Model file for the job. Use its own axes, mm. A direction names the side the tool comes from. Coordinates: 2 decimals unless noted, no trailing zeros. Order: outer loops, then holes, each group sorted by start corner. A loop starts at its lowest first (then second) coordinate and runs counter-clockwise, first axis right, second up. Notation, with made-up numbers: (57.5, 85) -> (66.5, 85) arc R28 ccw to (66.5, 103) -> close; hole circle Ø8 at (65, 8.5). An arc over 180 degrees is marked (long way). Write item = value, one per line. Start each with the question number.
Q1. 3-axis set-ups, long thin cutter, end or side, ignore diameter. For faces 4 (the face through (-48, -66.033, 6)), 5 (the face through (63, -53.033, 2)), 6 (the face through (66.033, 47, 6)): which of +Z, -Z, +X, -X, +Y, -Y reach the whole face in a straight line?
Q2. Flat gauge pins, fed straight in: pin 1 (6 mm diameter, centred on y = 32.5, z = 5, fed in from +X); pin 2 (2.5 mm diameter, centred on x = -61.5, z = 1.5, fed in from +Y); pin 3 (6.5 mm diameter, centred on x = 61.5, y = 61.5, fed in from -Z). Where does each tip first touch, or does it go through?
Q3. Cut at A-A, the plane y = -28. List the corners of the cut face in (x, z), plus the area to 3 significant figures.
Q4. Cut at B-B, the plane x = 50.5. List the corners of the cut face in (y, z), plus the area to 3 significant figures.
Q5. Mould opens along Y. For faces 1 (the face through (-63, -53.033, 2)), 2 (the face through (-66.033, -47, 6)), 3 (the face through (61.15, -62.06, 7.46)) say: +Y half, -Y half, draft (parallel to the pull), parting line (faces both ways), or undercut.
Q6. Cut at C-C, the plane z = 2. Give the number of separate pieces and of enclosed holes in the cut face, plus the area to 3 significant figures.
Q7. Wall check: line 1 (X direction, y = 57.5, z = 9); line 2 (X direction, y = 58, z = 6); line 3 (Y direction, x = 17.3, z = 3.5) (3 decimals). Give the ranges that are in metal, low to high. Write a range as from..to.
Autodesk Inventor part; units mm, degrees
ref_plane "YZ Plane" through (0, 0, 0) normal (1, 0, 0) x (0, 1, 0)
ref_plane "XZ Plane" through (0, 0, 0) normal (0, 1, 0) x (-1, 0, 0)
ref_plane "XY Plane" through (0, 0, 0) normal (0, 0, 1) x (1, 0, 0)
sketch "Эскиз1" plane through (0, 0, 0) normal (0, 0, 1) x (1, 0, 0)
  circle A0 centre (59.533, -59.533) radius 3
  circle A1 centre (-59.533, -59.533) radius 3
  circle A2 centre (-59.533, 59.533) radius 3
  circle A3 centre (59.533, 59.533) radius 3
  circle A4 centre (0, 0) radius 65
  arc A5 (35.5618, 66.033) -> (-35.5618, 66.033) centre (0, 0) ccw
  line L0 (-35.5618, 66.033) -> (-66.033, 66.033)
  line L1 (-66.033, 66.033) -> (-66.033, 35.5618)
  arc A6 (-66.033, 35.5618) -> (-66.033, -35.5618) centre (0, 0) ccw
  line L2 (-66.033, -35.5618) -> (-66.033, -66.033)
  line L3 (-66.033, -66.033) -> (-35.5618, -66.033)
  arc A7 (-35.5618, -66.033) -> (35.5618, -66.033) centre (0, 0) ccw
  line L4 (35.5618, -66.033) -> (66.033, -66.033)
  line L5 (66.033, -66.033) -> (66.033, -35.5618)
  arc A8 (66.033, -35.5618) -> (66.033, 35.5618) centre (0, 0) ccw
  line L6 (66.033, 35.5618) -> (66.033, 66.033)
  line L7 (66.033, 66.033) -> (35.5618, 66.033)
  point P0 (0, 0)
extrude "Выдавливание1" add sketch "Эскиз1" along normal blind 10 contours A4 | L7 L6 A8 L5 L4 A7 L3 L2 A6 L1 L0 A5
sketch "Эскиз8" plane through (0, 0, 0) normal (0, 0, -1) x (-1, 0, 0)
  arc A0 (-18, 26.5) -> (-26.5, 18) centre (-18, 18) ccw
  line L0 (-26.5, -18) -> (-26.5, 18)
  arc A1 (-26.5, -18) -> (-18, -26.5) centre (-18, -18) ccw
  line L1 (18, -26.5) -> (-18, -26.5)
  arc A2 (18, -26.5) -> (26.5, -18) centre (18, -18) ccw
  line L2 (26.5, 18) -> (26.5, -18)
  arc A3 (26.5, 18) -> (18, 26.5) centre (18, 18) ccw
  line L3 (-18, 26.5) -> (18, 26.5)
  circle A4 centre (-21.2132, 21.2132) radius 1.5
  circle A5 centre (-21.2132, -21.2132) radius 1.5
  circle A6 centre (21.2132, -21.2132) radius 1.5
  circle A7 centre (21.2132, 21.2132) radius 1.5
  circle A8 centre (0, 0) radius 22
extrude "Выдавливание6" cut sketch "Эскиз8" against normal blind 10 contours A4 | A5 | A6 | A7
sketch "Эскиз9" plane through (0, 0, 0) normal (0, 0, -1) x (-1, 0, 0)
  line L0 (20.1, -44.6) -> (20.1, 8.5)
  line L1 (20.1, 8.5) -> (15, 14.5)
  line L2 (11.5, 14.5) -> (15, 14.5)
  line L3 (11.5, 14.5) -> (-11.5, 14.5)
  line L4 (-15, 14.5) -> (-11.5, 14.5)
  line L5 (-15, 14.5) -> (-20.1, 8.5)
  line L6 (-20.1, 8.5) -> (-20.1, -44.6)
  line L7 (-20.1, -44.6) -> (-15, -50.6)
  line L8 (-15, -50.6) -> (15, -50.6)
  line L9 (15, -50.6) -> (20.1, -44.6)
  circle A0 centre (11, -47.8) radius 1.025
  circle A1 centre (-11, -47.8) radius 1.025
  circle A2 centre (-17.3, -40) radius 1.025
  circle A3 centre (17.3, -40) radius 1.025
  circle A4 centre (17.3, -18) radius 1.025
  circle A5 centre (17.3, 4) radius 1.025
  circle A6 centre (-17.3, 4) radius 1.025
  circle A7 centre (0, 0) radius 1.55
  circle A8 centre (0, 0) radius 14
  line L10 (-14.5, 11.5) -> (-14.5, -42)
  arc A9 (-11.5, 14.5) -> (-14.5, 11.5) centre (-11.5, 11.5) ccw
  arc A10 (-14.5, -42) -> (-11.5, -45) centre (-11.5, -42) ccw
  line L11 (-20.1, 8.5) -> (-20.1, -44.6)
  arc A11 (14.5, 11.5) -> (11.5, 14.5) centre (11.5, 11.5) ccw
  line L12 (14.5, -42) -> (14.5, 11.5)
  arc A12 (11.5, -45) -> (14.5, -42) centre (11.5, -42) ccw
  line L13 (-11.5, -45) -> (11.5, -45)
  circle A13 centre (-17.3, -18) radius 1.025
extrude "Выдавливание7" cut sketch "Эскиз9" against normal blind 20.75 contours A11 L12 A12 L13 A10 L10 A9 L3 | A0 | A1 | A2 | A3 | A4 | A5 | A6 | A7 | A8 | A13
sketch "Эскиз10" plane through (0, 0, 0) normal (0, 0, -1) x (-1, 0, 0)
  circle A0 centre (59.533, -59.533) radius 3
  circle A1 centre (59.533, -59.533) radius 6.5
  line L0 (66.033, -66.033) -> (35.5618, -66.033)
  line L1 (66.033, -35.5618) -> (66.033, -66.033)
  line L2 (59.533, -53.033) -> (66.033, -53.033)
  line L3 (66.033, -53.033) -> (66.033, -66.033)
  line L4 (66.033, -66.033) -> (53.033, -66.033)
  line L5 (53.033, -66.033) -> (53.033, -59.533)
  point P0 (0, 0)
extrude "Выдавливание8" cut sketch "Эскиз10" against normal blind 5
pattern_circular "Круговой массив1" count 4 over 360 about axis through (0, 0, 0) along (0, 0, 1) of "Выдавливание8"
properties part number "000.202 - Крышка" material "Пластик АБС"
Here are the results:
q1.face_4 = +Z, -Z, -X, -Y
q1.face_5 = -Z, +X, -Y
q1.face_6 = +Z, -Z, +X, +Y
q2.pin_1 = 68.95
q2.pin_2 = 53.03
q2.pin_3 = 5
q3.outline = (-69.58, 0) -> (-14.5, 0) -> (-14.5, 10) -> (-69.58, 10) -> close; (14.5, 0) -> (69.58, 0) -> (69.58, 10) -> (14.5, 10) -> close
q3.area = 1,100 mm²
q4.outline = (-66.03, 0) -> (66.03, 0) -> (66.03, 10) -> (-66.03, 10) -> close
q4.area = 1,320 mm²
q5.face_1 = -Y half
q5.face_2 = draft
q5.face_3 = undercut
q6.separate_pieces = 1
q6.enclosed_holes = 13
q6.area = 16,800 mm²
q7.line_1 = -66.03..-61.74, -57.33..57.33, 61.74..66.03
q7.line_2 = -66.03..-62.11, -56.95..56.95, 62.11..66.03
q7.line_3 = -72.977..-41.025, -38.975..-19.025, -16.975..2.975, 5.025..72.977
